Geometry check sheet. Reference: the model listing, model coordinates, mm. A direction names the side the tool comes from. Give positions to 0.01 mm unless a question says otherwise; leave off trailing zeros. Loops run counter-clockwise (first coordinate to the right, second up) from the corner with the lowest first, then second, coordinate; pieces in that order, holes last. Notation, with made-up numbers: (-24.75, 12.5) - (7.25, 12.5) arc R20 ccw to (7.25, 33.5) - close; hole circle Ø2 at (69.5, -26.5). An arc over 180 degrees is marked (long way). Write item = value, one per line. Start each with the question number.
Autodesk Inventor part; units mm, degrees
ref_plane "YZ Plane" through (0, 0, 0) normal (1, 0, 0) x (0, 1, 0)
ref_plane "XZ Plane" through (0, 0, 0) normal (0, 1, 0) x (-1, 0, 0)
ref_plane "XY Plane" through (0, 0, 0) normal (0, 0, 1) x (1, 0, 0)
sketch "Náčrt1" plane through (0, 0, 0) normal (0, 0, 1) x (1, 0, 0)
  line L0 (-29, -47) -> (29, -47)
  line L1 (29, -47) -> (29, 47)
  line L2 (29, 47) -> (-29, 47)
  line L3 (-29, 47) -> (-29, -47)
  line L4 (-29, -47) -> (29, 47) construction
  line L5 (29, -47) -> (-29, 47) construction
  line L6 (0, 47) -> (0, -47)
  line L7 (0, -43.9165) -> (12.5, -43.9165)
  point P0 (0, 0)
  dimension "d0" = 58
  dimension "d1" = 94
  dimension "d2" = 12.5
extrude "Vysunutí1" add sketch "Náčrt1" along normal blind 3
sketch "Náčrt2" plane through (0, 0, 3) normal (0, 0, 1) x (1, 0, 0)
  point P0 (0, 0)
sketch "Náčrt3" plane through (0, 0, 3) normal (0, 0, 1) x (1, 0, 0)
  line L0 (0, -40.9336) -> (12.5, -40.9336)
  circle A0 centre (12.5, -40.9336) radius 1.45
  line L1 (0, 0) -> (0, -12.3388)
  circle A1 centre (-12.5, -40.9336) radius 1.45
  line L2 (-12.5, -39.4836) -> (-12.5, 38.0164)
  circle A2 centre (-12.5, 39.5164) radius 1.45
  circle A3 centre (12.5, 39.5164) radius 1.45
  dimension "d5" = 12.5
  dimension "d6" = 2.9
  dimension "d7" = 77.5
  dimension "d8" = 2.9
  dimension "d9" = 1.5
extrude "Vysunutí2" add sketch "Náčrt3" along normal blind 12
sketch "Náčrt4" plane through (0, 0, 3) normal (0, 0, 1) x (1, 0, 0)
  circle A0 centre (12.5, 39.5164) radius 1.45
  circle A1 centre (12.5, 39.5164) radius 2.5
  circle A2 centre (-12.5, 39.5164) radius 1.45
  circle A3 centre (-12.5, 39.5164) radius 2.5
  circle A4 centre (-12.5, -40.9336) radius 1.45
  circle A5 centre (-12.5, -40.9336) radius 2.5
  circle A6 centre (12.5, -40.9336) radius 1.45
  circle A7 centre (12.5, -40.9336) radius 2.5
  point P0 (0, 0)
  dimension "d12" = 5
  dimension "d13" = 5
  dimension "d14" = 5
  dimension "d15" = 5
extrude "Vysunutí3" add sketch "Náčrt4" along normal blind 8 contours A0 | A1 | A2 | A3 | A4 | A5 | A6 | A7
properties part number "drzak_plos"
1) Tool access check on faces 1 (the face through (-13, -41, 15)), 2 (the face through (11.05, -41, 12.97)). Record the directions out of +Z, -Z, +X, -X, +Y, -Y that give a thin tool (end or side, any length) a straight path to the whole face; none if there is none.
2) Material ranges on line 1 along Z through (x, y) = (11, 35); line 2 along X through (y, z) = (40.5, 10); line 3 along X through (y, z) = (38, 10.5), recorded low to high.
3) Cross-section at D-D on x = 13. Enter the section's corners in (y, z), and give its area (3 significant figures).
4) Cross-section at C-C on y = -8. Enter the section's corners in (x, z).
5) Gauge pin test, flat ends, axial feed: P1, Ø6, axis at x = 17.5, z = 12, coming from the -Y side; P2, Ø2, axis at x = -11, y = 20.5, coming from the +Z side; P3, Ø2, axis at y = 37.5, z = 11.5, coming from the -X side; P4, Ø5, axis at x = -18.5, y = 19, coming from the -Z side. Record the tip position at first contact, or that the pin passes through.
6) Cross-section at B-B on z = 6.75. Enter the section's corners in (x, y).
7) Cross-section at A-A on x = -12.5. Enter the section's corners in (y, z).
8) Release check for a two-part mould opening along Y. For faces 3 (the face through (0, 47, 1)), 4 (the face through (-29, 1, 1)), 5 (the face through (14, 38, 11)) record: pulls with the +Y half, pulls with the -Y half, needs draft (parallel to the pull), parting line crosses it, or undercut.
Checked values:
q1.face_1 = +Z, +X, -X, +Y, -Y
q1.face_2 = +Z
q2.line_1 = 0 to 3
q2.line_2 = -14.8 to -10.2, 10.2 to 14.8
q2.line_3 = -14.49 to -10.51, 10.51 to 14.49
q3.outline = (-47, 0) - (47, 0) - (47, 3) - (41.97, 3) - (41.97, 11) - (40.88, 11) - (40.88, 15) - (38.16, 15) - (38.16, 11) - (37.07, 11) - (37.07, 3) - (-38.48, 3) - (-38.48, 11) - (-39.57, 11) - (-39.57, 15) - (-42.29, 15) - (-42.29, 11) - (-43.38, 11) - (-43.38, 3) - (-47, 3) - close
q3.area = 382 mm²
q4.outline = (-29, 0) - (29, 0) - (29, 3) - (-29, 3) - close
q5.P1 = -42.17
q5.P2 = 3
q5.P3 = -14.72
q5.P4 = 0
q6.outline = circle Ø5 at (-12.5, -40.93); circle Ø5 at (-12.5, 39.52); circle Ø5 at (12.5, -40.93); circle Ø5 at (12.5, 39.52)
q7.outline = (-47, 0) - (47, 0) - (47, 3) - (42.02, 3) - (42.02, 11) - (40.97, 11) - (40.97, 15) - (38.07, 15) - (38.07, 11) - (37.02, 11) - (37.02, 3) - (-38.43, 3) - (-38.43, 11) - (-39.48, 11) - (-39.48, 15) - (-42.38, 15) - (-42.38, 11) - (-43.43, 11) - (-43.43, 3) - (-47, 3) - close
q8.face_3 = pulls with the +Y half
q8.face_4 = needs draft
q8.face_5 = undercut
